from build123d import *

# Parameters (mm, degrees)
SKETCH1_W                  = 22.225
SKETCH1_H                  = 22.225
BOSS_EXTRUDE1_DEPTH        = 44.45
M10X1_5_TAPPED_HOLE1_D     = 8.5
M10X1_5_TAPPED_HOLE1_DEPTH = 24.638
M10X1_5_TAPPED_HOLE1_TIP   = 2.553657631
SKETCH9_R                  = 4.25
CUT_EXTRUDE1_DEPTH         = 19.05
SKETCH10_R                 = 7.14375
CUT_EXTRUDE2_DEPTH         = 9.525
SKETCH11_R                 = 1.984375
CUT_EXTRUDE3_DEPTH         = 23.225
SKETCH12_R                 = 1.984375
CUT_EXTRUDE4_DEPTH         = 23.225


with BuildPart() as part:
    # Sketch1 → Boss-Extrude1 (new body)
    with BuildSketch(Plane(origin=(0, 0, 0), x_dir=(1, 0, 0), z_dir=(0, 1, 0))):
        Rectangle(SKETCH1_W, SKETCH1_H)
    extrude(amount=BOSS_EXTRUDE1_DEPTH)

    # M10x1.5 Tapped Hole1
    with Locations(Plane(origin=(0, 0, 0), x_dir=(-1, 0, 0), z_dir=(0, -1, 0))):
        with Locations((0, 0)):
            Hole(M10X1_5_TAPPED_HOLE1_D / 2, depth=M10X1_5_TAPPED_HOLE1_DEPTH)
            with Locations((0, 0, -(M10X1_5_TAPPED_HOLE1_DEPTH + M10X1_5_TAPPED_HOLE1_TIP / 2))):  # 118° drill point
                Cone(0, M10X1_5_TAPPED_HOLE1_D / 2, M10X1_5_TAPPED_HOLE1_TIP, mode=Mode.SUBTRACT)

    # Sketch9 → Cut-Extrude1 (cut)
    with BuildSketch(Plane(origin=(0, 44.45, 0), x_dir=(1, 0, 0), z_dir=(0, 1, 0))):
        Circle(SKETCH9_R)
    extrude(amount=-CUT_EXTRUDE1_DEPTH, mode=Mode.SUBTRACT)

    # Sketch10 → Cut-Extrude2 (cut)
    with BuildSketch(Plane(origin=(0, 44.45, 0), x_dir=(1, 0, 0), z_dir=(0, 1, 0))):
        Circle(SKETCH10_R)
    extrude(amount=-CUT_EXTRUDE2_DEPTH, mode=Mode.SUBTRACT)

    # Sketch11 → Cut-Extrude3 (cut, through all)
    with BuildSketch(Plane(origin=(11.1125, 0, 0), x_dir=(0, 0, -1), z_dir=(1, 0, 0))):
        with Locations((0, 31.75)):
            Circle(SKETCH11_R)
    extrude(amount=-CUT_EXTRUDE3_DEPTH, mode=Mode.SUBTRACT)

    # Sketch12 → Cut-Extrude4 (cut, through all)
    with BuildSketch(Plane.XY.offset(11.1125)):
        with Locations((0, 31.75)):
            Circle(SKETCH12_R)
    extrude(amount=-CUT_EXTRUDE4_DEPTH, mode=Mode.SUBTRACT)


solid = part.part
The listing builds one solid part. Answer for the finished solid, in the listing's coordinates (mm). A direction names the side the tool comes from. Round coordinates to 2 decimals unless told otherwise and drop trailing zeros. Order: outer loops, then holes, each group sorted by start corner. A loop starts at its lowest first (then second) coordinate and runs counter-clockwise, first axis right, second up. Notation, with made-up numbers: (66, -9) -> (79, -9) arc R7 cw to (79, -1) -> close; hole circle Ø7 at (27, -36). An arc over 180 degrees is marked (long way). Write each question's results on one line, items separated by ' | '. Start each with the question number.
Q1. Each of these flat-tipped pins is pushed along its axis until it touches: pin 1 (7 mm diameter, centred on x = 1.5, z = 0.5, fed in from +Y) (3 decimals); pin 2 (7 mm diameter, centred on x = 0, z = 0, fed in from -Y). Where does it stop, or does it pass through?
Q2. Straight lines are drawn through the part: probe 1 along X at (y, z) = (41, 0); probe 2 along Y at (x, z) = (-9.5, 0); probe 3 along Z at (x, y) = (-6.75, 31.75). For each, find the intervals that lie inside material, in ascending order. Write a range as from..to.
Q3. Find section B-B (x = 0). Give the number of separate pieces and of enclosed holes in the cut face, then the cut area to 3 significant figures.
Q4. Find section A-A (y = 31.75). Determine the outline of the cut face in (x, z).
Q5. The mould has two halves that part along X. Classify faces 4 (the flat face through (0, 22, -11.112)), 5 (the flat face through (11.112, 22, 0)), 6 (the flat face through (0, 34.925, 5)): pulls with the +X half, pulls with the -X half, needs draft (parallel to the pull), parting line crosses it, or undercut.
Q6. Find section D-D (y = 15). Determine the outline of the cut face in (x, z).
Q7. Which of the six approach directions +Z, -Z, +X, -X, +Y, -Y give full straight-line access (tool end or side, diameter ignored) to faces 1 (the flat face through (2, 25.4, 3)), 2 (the flat face through (5, 0, 0)), 3 (the cylindrical face through (2.285, 12.491, -3.584))?
Worked answers:
1) pin 1: stops at y = 34.925 | pin 2: stops at y = 25.09
2) probe 1: x = -11.11..-7.14, 7.14..11.11 | probe 2: y = 0..29.77, 33.73..44.45 | probe 3: z = -11.11..-1.98, 1.98..11.11
3) separate pieces: 4 | enclosed holes: 0 | area: 501 mm2
4) outline: (-11.11, -11.11) -> (-1.98, -11.11) -> (-1.98, -3.76) arc R4.25 cw to (-3.76, -1.98) -> (-11.11, -1.98) -> close; (-11.11, 1.98) -> (-3.76, 1.98) arc R4.25 cw to (-1.98, 3.76) -> (-1.98, 11.11) -> (-11.11, 11.11) -> close; (1.98, -11.11) -> (11.11, -11.11) -> (11.11, -1.98) -> (3.76, -1.98) arc R4.25 cw to (1.98, -3.76) -> close; (1.98, 3.76) arc R4.25 cw to (3.76, 1.98) -> (11.11, 1.98) -> (11.11, 11.11) -> (1.98, 11.11) -> close
5) face 4: needs draft | face 5: pulls with the +X half | face 6: undercut
6) outline: (-11.11, -11.11) -> (11.11, -11.11) -> (11.11, 11.11) -> (-11.11, 11.11) -> close; hole circle Ø8.5 at (0, 0)
7) face 1: +Y | face 2: +Z, -Z, +X, -X, -Y | face 3: -Y
